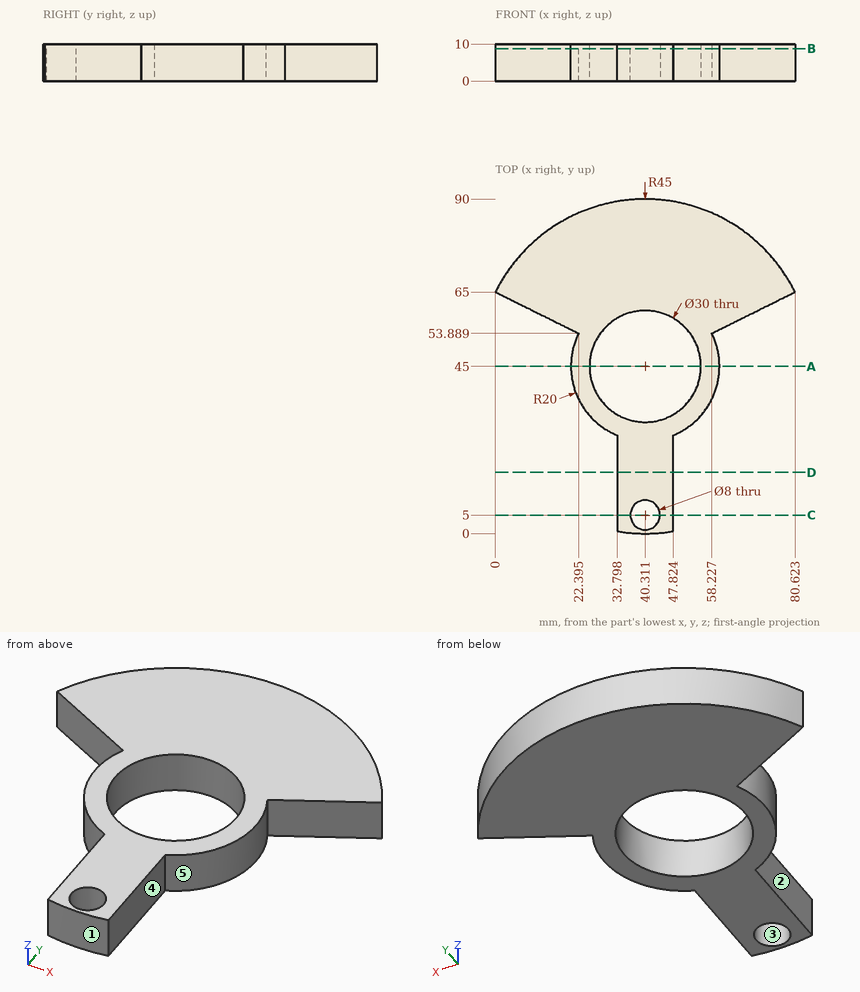
The drawing under review shows one solid part. Ordinate dimensions are in mm from its lowest x, y, z. A direction names the side the tool comes from. Round coordinates to 2 decimals unless told otherwise and drop trailing zeros. Write each loop counter-clockwise with the first axis right and the second up, starting at its lowest first coordinate (ties: lowest second). Pieces come first, ordered by that corner, then holes. Notation, with made-up numbers: M 7,19.25 L 43,19.25 A33 cw 43,55.25 Z; hole C 68,-37 d11. An arc over 180 degrees is marked long. One line per item, written item: value. Start each with the question number.
(1) Wall thickness on line 1 (Y direction, x = 39.5, z = 7.5); line 2 (Y direction, x = 37, z = 4.5) (1 decimal); line 3 (X direction, y = 16, z = 6) (1 decimal): over which ranges is each line inside the solid? List them lowest first.
(2) The part is to be moulded in two halves that separate along Y. For the marked faces 1, 2 and 3, say which applies: released by +Y, released by -Y, zero draft, split by the parting line, or undercut.
(3) We need section B-B (z = 8.75). Give the boundary of the cut face in (x, y) (1 decimal).
(4) We need section A-A (y = 45). Give the boundary of the cut face in (x, z), and give its area (3 significant figures).
(5) Insertion check: pin 1 (4 mm diameter, centred on y = 20, z = 5.5, fed in from -X); pin 2 (6 mm diameter, centred on x = 32, y = 60, fed in from -Z); pin 3 (1 mm diameter, centred on x = 22.5, z = 4.5, fed in from -Y) (1 decimal); pin 4 (4 mm diameter, centred on x = 23, z = 6, fed in from +Y) (1 decimal). Each pin has a flat end and moves straight along its axis. Give the tip position at first contact, or say it passes through.
(6) We need section C-C (y = 5). Give the boundary of the cut face in (x, z) (1 decimal).
(7) Machinability: for the marked faces 4 and 5, which of the approach directions +Z, -Z, +X, -X, +Y, -Y give a long, thin tool a straight path to every point of the face, cutting with its end or side? Answer none if there is none.
(8) We need section D-D (y = 16.5). Give the boundary of the cut face in (x, z) (1 decimal).
Result:
1. line 1: 0.01 to 1.08, 8.92 to 30.02, 59.98 to 89.99
1. line 2: 0.1 to 2.8, 7.2 to 30.4, 59.6 to 89.9
1. line 3: 32.8 to 47.8
2. face 1: released by -Y
2. face 2: zero draft
2. face 3: undercut
3. outline: M 0,65 L 22.4,53.9 A20 ccw 32.8,26.5 L 32.8,0.6 A45 ccw 47.8,0.6 L 47.8,26.5 A20 ccw 58.2,53.9 L 80.6,65 A45 ccw Z; hole C 40.3,45 d30; hole C 40.3,5 d8
4. outline: M 20.31,0 L 25.31,0 L 25.31,10 L 20.31,10 Z; M 55.31,0 L 60.31,0 L 60.31,10 L 55.31,10 Z
4. area: 100 mm²
5. pin 1: x = 32.8
5. pin 2: z = 0
5. pin 3: y = 35
5. pin 4: y = 87.3
6. outline: M 32.8,0 L 36.3,0 L 36.3,10 L 32.8,10 Z; M 44.3,0 L 47.8,0 L 47.8,10 L 44.3,10 Z
7. face 4: +Z, -Z, +X, -Y
7. face 5: +Z, -Z, +X
8. outline: M 32.8,0 L 47.8,0 L 47.8,10 L 32.8,10 Z
